from build123d import *

# Parameters (mm, degrees)
SKETCH1_W           = 309.88
SKETCH1_H           = 136.398
BOSS_EXTRUDE1_DEPTH = 160.528
SKETCH2_R           = 19.05
BOSS_EXTRUDE2_DEPTH = 56.896
SKETCH3_R           = 34.925
BOSS_EXTRUDE3_DEPTH = 12.7


with BuildPart() as part:
    # Sketch1 → Boss-Extrude1 (new body)
    with BuildSketch(Plane.XY):
        with Locations((111.640327538, -47.419508944)):
            Rectangle(SKETCH1_W, SKETCH1_H)
    extrude(amount=BOSS_EXTRUDE1_DEPTH)

    # Sketch2 → Boss-Extrude2 (add)
    with BuildSketch(Plane.XY.offset(160.528)):
        with Locations((111.640327538, -47.419508944)):
            Circle(SKETCH2_R)
    extrude(amount=BOSS_EXTRUDE2_DEPTH)

    # Sketch3 → Boss-Extrude3 (add)
    with BuildSketch(Plane.XY.offset(217.424)):
        with Locations((111.640327538, -47.419508944)):
            Circle(SKETCH3_R)
    extrude(amount=BOSS_EXTRUDE3_DEPTH)


solid = part.part
The listing builds one solid part. Answer for the finished solid, in the listing's coordinates (mm). A direction names the side the tool comes from. Round coordinates to 2 decimals unless told otherwise and drop trailing zeros. Order: outer loops, then holes, each group sorted by start corner. A loop starts at its lowest first (then second) coordinate and runs counter-clockwise, first axis right, second up. Notation, with made-up numbers: (42, 48.5) -> (59, 48.5) arc R26 cw to (59, 67.5) -> close; hole circle Ø4 at (4.5, 34). An arc over 180 degrees is marked (long way). One line per item, written item: value.
Item 1: For a pull along Z with two mould halves and no side action, classify faces 1 (the cylindrical face through (76.75, -45.88, 223.69)), 2 (the flat face through (127, -62, 217.424)), 3 (the flat face through (111, -47, 230.124)) as released by +Z, released by -Z, zero draft, split by the parting line, or undercut.
Taken from the geometry:
face 1: zero draft
face 2: undercut
face 3: released by +Z
Item 2: Find section C-C, the plane y = 4. Give the vertices of the cut face in (x, z), then the cut area to 3 significant figures.
Taken from the geometry:
outline: (-43.3, 0) -> (266.58, 0) -> (266.58, 160.53) -> (-43.3, 160.53) -> close
area: 49,700 mm2
Item 3: For faces 4 (the flat face through (266.58, -48, 79)), 5 (the cylindrical face through (92.61, -46.58, 188.58)), determine the directions among +Z, -Z, +X, -X, +Y, -Y from which every point of the face is accessible in a straight line to the end or side of a thin tool.
Taken from the geometry:
face 4: +Z, -Z, +X, +Y, -Y
face 5: none
Item 4: Find section D-D, the plane x = 126. Give the vertices of the cut face in (y, z).
Taken from the geometry:
outline: (-115.62, 0) -> (20.78, 0) -> (20.78, 160.53) -> (-34.9, 160.53) -> (-34.9, 217.42) -> (-15.58, 217.42) -> (-15.58, 230.12) -> (-79.26, 230.12) -> (-79.26, 217.42) -> (-59.94, 217.42) -> (-59.94, 160.53) -> (-115.62, 160.53) -> close
Item 5: Find section B-B, the plane x = 84. Give the vertices of the cut face in (y, z).
Taken from the geometry:
outline: (-115.62, 0) -> (20.78, 0) -> (20.78, 160.53) -> (-115.62, 160.53) -> close; (-68.77, 217.42) -> (-26.07, 217.42) -> (-26.07, 230.12) -> (-68.77, 230.12) -> close
Item 6: Straight lines are drawn through the part: L1, parallel to Z at x = 86.5, y = -54; L2, parallel to Z at x = 155, y = -59; L3, parallel to X at y = -57.5, z = 185. For each, find the intervals that lie inside material, in ascending order.
Taken from the geometry:
L1: z = 0 to 160.53, 217.42 to 230.12
L2: z = 0 to 160.53
L3: x = 95.48 to 127.8
Item 7: Find section A-A, the plane y = -17. Give the vertices of the cut face in (x, z).
Taken from the geometry:
outline: (-43.3, 0) -> (266.58, 0) -> (266.58, 160.53) -> (-43.3, 160.53) -> close; (94.48, 217.42) -> (128.8, 217.42) -> (128.8, 230.12) -> (94.48, 230.12) -> close
